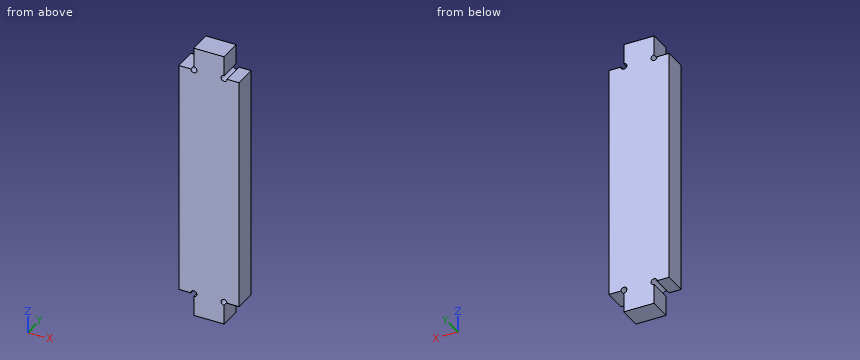
```python
from build123d import *

# Parameters (mm, degrees)
BOSS_EXTRUDE2_DEPTH = 3
CUT_EXTRUDE5_DEPTH  = 3


with BuildPart() as part:
    # Sketch1 → Boss-Extrude2 (new body)
    with BuildSketch(Plane(origin=(0, 0, 0), x_dir=(1, 0, 0), z_dir=(0, 1, 0))):
        Polygon((4, 15.5), (4, -15.5), (2, -15.5), (2, -18.5), (-2, -18.5), (-2, -15.5), (-4, -15.5), (-4, 15.5), (-2, 15.5), (-2, 18.5), (2, 18.5), (2, 15.5), align=None)
    extrude(amount=BOSS_EXTRUDE2_DEPTH)

    # Sketch4 → Cut-Extrude5 (cut)
    with BuildSketch(Plane(origin=(0, 3, 0), x_dir=(1, 0, 0), z_dir=(0, 1, 0))):
        with BuildLine():
            Line((2, 15.9), (2, 15.5))
            Line((2, 15.5), (2.4, 15.5))
            ThreePointArc((2.4, 15.5), (1.717157288, 15.217157288), (2, 15.9))
        make_face()
        with BuildLine():
            Line((-2, 15.5), (-2.4, 15.5))
            ThreePointArc((-2.4, 15.5), (-1.717157288, 15.217157288), (-2, 15.9))
            Line((-2, 15.9), (-2, 15.5))
        make_face()
        with BuildLine():
            Line((-2, -15.9), (-2, -15.5))
            Line((-2, -15.5), (-2.4, -15.5))
            ThreePointArc((-2.4, -15.5), (-1.717157288, -15.217157288), (-2, -15.9))
        make_face()
        with BuildLine():
            Line((2, -15.5), (2.4, -15.5))
            ThreePointArc((2.4, -15.5), (1.717157288, -15.217157288), (2, -15.9))
            Line((2, -15.9), (2, -15.5))
        make_face()
    extrude(amount=-CUT_EXTRUDE5_DEPTH, mode=Mode.SUBTRACT)


solid = part.part
```
Design review of the part built by this model. Coordinates are the model's own, in mm. Give positions to 0.01 mm unless a question says otherwise; leave off trailing zeros. Order: outer loops, then holes, each group sorted by start corner. A loop starts at its lowest first (then second) coordinate and runs counter-clockwise, first axis right, second up. Notation, with made-up numbers: (59.5, -8) -> (89.5, -8) arc R12 ccw to (89.5, 11) -> close; hole circle Ø10 at (21, -8). An arc over 180 degrees is marked (long way). Write item = value, one per line. Start each with the question number.
(1) We need section B-B on x = -3. Write out the cut boundary in (y, z).
(2) For pin 1 (0.5 mm diameter, centred on x = -3, y = 1.5, fed in from -Z); pin 2 (0.8 mm diameter, centred on y = 1.5, z = 17.5, fed in from +X); pin 3 (0.8 mm diameter, centred on x = -3.5, y = 1.5, fed in from +Z), all flat-tipped, find the tip position at first contact; note any pin that passes through.
(3) To check wall thickness, follow line 1 along Z through (x, y) = (-1.75, 2.85); line 2 along Z through (x, y) = (-3.25, 1.7). State the ranges of each line that lie inside material, in increasing order.
(4) We need section A-A on y = 1.6. Write out the cut boundary in (x, z).
Numbers:
q1.outline = (0, -15.5) -> (3, -15.5) -> (3, 15.5) -> (0, 15.5) -> close
q2.pin_1 = -15.5
q2.pin_2 = 2
q2.pin_3 = 15.5
q3.line_1 = -18.5 to -15.81, -15.19 to 15.19, 15.81 to 18.5
q3.line_2 = -15.5 to 15.5
q4.outline = (-4, -15.5) -> (-2.4, -15.5) arc R0.4 cw (long way) to (-2, -15.9) -> (-2, -18.5) -> (2, -18.5) -> (2, -15.9) arc R0.4 cw (long way) to (2.4, -15.5) -> (4, -15.5) -> (4, 15.5) -> (2.4, 15.5) arc R0.4 cw (long way) to (2, 15.9) -> (2, 18.5) -> (-2, 18.5) -> (-2, 15.9) arc R0.4 cw (long way) to (-2.4, 15.5) -> (-4, 15.5) -> close
